Input: part model. Units: mm. Frame: model coordinates. Face numbers are marked on the shaded views. Round coordinates to 2 decimals unless told otherwise and drop trailing zeros. Order: outer loops, then holes, each group sorted by start corner. A loop starts at its lowest first (then second) coordinate and runs counter-clockwise, first axis right, second up.
Item 1: Line query: L1, parallel to Z at x = -51.5, y = 24.5; L2, parallel to Y at x = -21.5, z = 17; L3, parallel to Y at x = 32, z = 23. Output: solid intervals per line, ascending.
Item 2: Mould query, pull axis Y, two halves, no side actions, for the marked faces 1 and 2. Classes: released by +Y, released by -Y, zero draft, split by the parting line, or undercut.
Item 3: Cut plane B-B on y = 5.5. Output: boundary loops of the cut face in (x, z).
Item 4: Cut plane D-D on y = 37. Output: boundary loops of the cut face in (x, z), then the cut area to 3 significant figures.
Item 5: Cut plane A-A on z = -4. Output: boundary loops of the cut face in (x, y), then the cut area to 3 significant figures.
Item 6: First-contact query: pin 1 (1.5 mm diameter, centred on x = 27.5, z = 4.5, fed in from +Y); pin 2 (10 mm diameter, centred on x = -39, z = 19, fed in from +Y); pin 3 (2 mm diameter, centred on y = 35.5, z = 17.5, fed in from +X). Flat tips, straight axial feed; report the tip coordinate or a pass-through.
Item 7: Cut plane C-C on x = -40.5. Output: boundary loops of the cut face in (y, z).
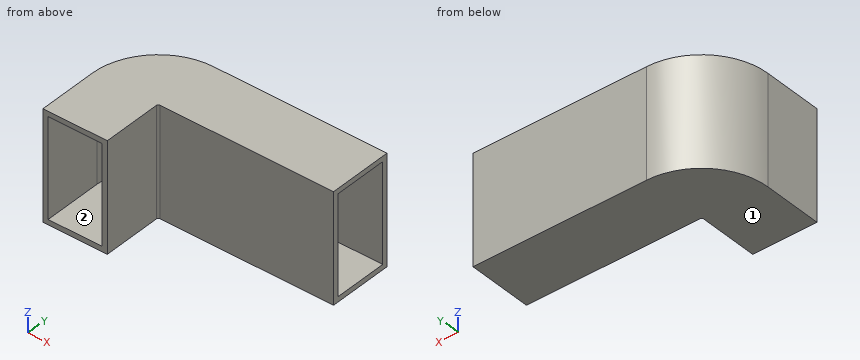
```python
from build123d import *

# Parameters (mm, degrees)
SKETCH2_W   = 63.80012688
SKETCH2_H   = 37.602651942
SKETCH2_W_2 = 57.80012688
SKETCH2_H_2 = 31.602651942


with BuildPart() as part:
    # Sweep-Thin1: sweep along a path in Sketch1
    with BuildLine(Plane.XY) as sweep_thin1_path:
        Line((-43.035286794, -24.171802054), (-44.234672924, 10.250579859))
        ThreePointArc((-44.234672924, 10.250579859), (-38.872819675, 24.588121657), (-24.943243853, 30.934891896))
        Line((-24.943243853, 30.934891896), (76.426266413, 34.466930581))
    # Sketch2 → Sweep-Thin1 (sweep)
    with BuildSketch(Plane(origin=(76.426266413, 34.466930581, 0), x_dir=(0, 0, -1), z_dir=(0.999393527672129, 0.034822074134917426, 0))):
        Rectangle(SKETCH2_W, SKETCH2_H)
        Rectangle(SKETCH2_W_2, SKETCH2_H_2, mode=Mode.SUBTRACT)
    sweep(path=sweep_thin1_path.line)


solid = part.part
```
From the geometry:
1. L1: z = -31.9 to -28.9, 28.9 to 31.9
1. L2: y = 12.24 to 15.24, 46.87 to 49.87
1. L3: y = 14.11 to 17.11, 48.73 to 51.73
2. face 1: zero draft
2. face 2: undercut
3. outline: (-62.88, -31.9) - (-25.26, -31.9) - (-25.26, 31.9) - (-62.88, 31.9) - close; hole (-59.88, -28.9) - (-28.26, -28.9) - (-28.26, 28.9) - (-59.88, 28.9) - close
4. outline: (-53, -31.9) - (76.34, -31.9) - (76.34, -28.9) - (-48.8, -28.9) - (-48.8, 28.9) - (76.34, 28.9) - (76.34, 31.9) - (-53, 31.9) - close
4. area: 1,020 mm2
5. outline: (-63.02, 9.6) - (-61.83, -24.83) - (-58.83, -24.72) - (-60.03, 9.7) arc R35.8 cw to (-25.49, 46.73) - (75.88, 50.26) - (75.77, 53.26) - (-25.6, 49.72) arc R38.8 ccw to start; (-28.44, 10.8) - (-27.24, -23.62) - (-24.25, -23.52) - (-25.44, 10.91) arc R1.2 cw to (-24.29, 12.14) - (77.08, 15.68) - (76.98, 18.68) - (-24.39, 15.14) arc R4.2 ccw to start
5. area: 1,000 mm2
6. pin 1: stops at y = 51.6
6. pin 2: stops at y = 48.5
6. pin 3: stops at x = -49.32
7. outline: (-24.08, -31.9) - (46.18, -31.9) - (46.18, 31.9) - (-24.08, 31.9) - (-24.08, 28.9) - (42.85, 28.9) - (42.85, -28.9) - (-24.08, -28.9) - close
